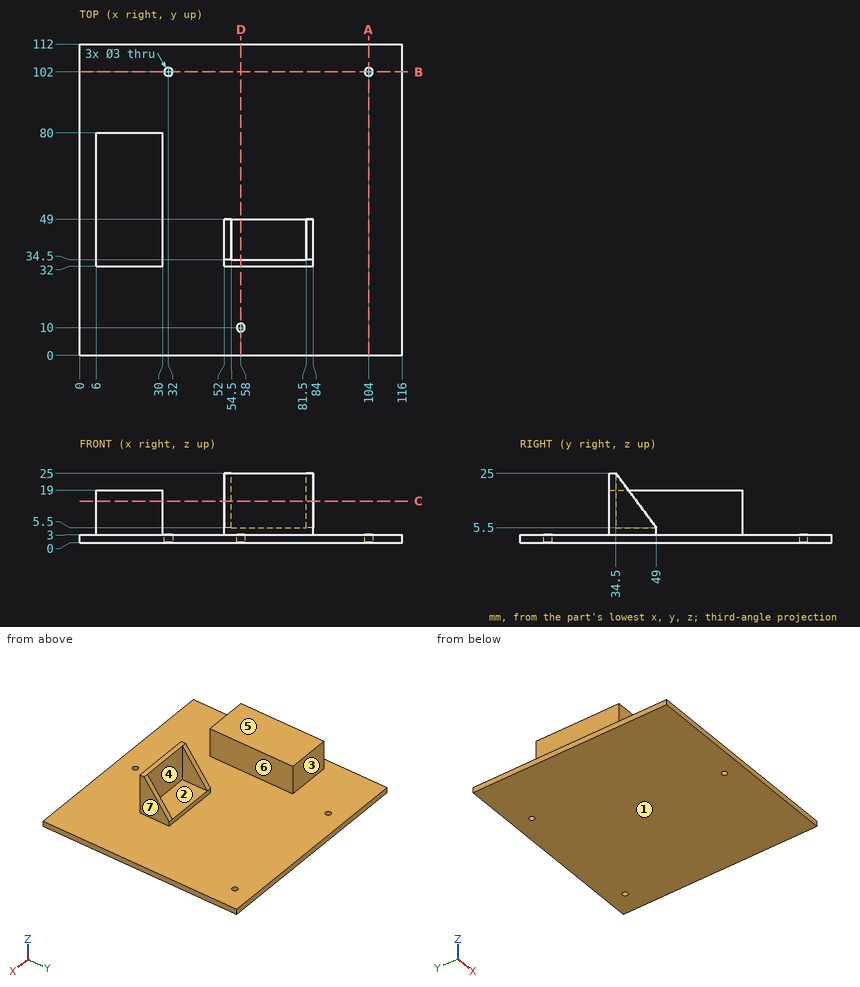
Study the drawing (mm; zero at the part's minimum x, y, z) and answer. A direction names the side the tool comes from. Give positions to 0.01 mm unless a question says otherwise; leave off trailing zeros. Write each loop counter-clockwise with the first axis right and the second up, starting at its lowest first coordinate (ties: lowest second). Pieces come first, ordered by that corner, then holes.
Item 1: Section A-A, the plane x = 104 is taken. Write down the section's boundary in (y, z).
Item 2: Section C-C, the plane z = 15 is taken. Write down the section's boundary in (x, y), plus the area to 3 significant figures.
Item 3: Section D-D, the plane x = 58 is taken. Write down the section's boundary in (y, z).
Item 4: Determine the mould class of the marked faces 4, 5, 6 and 7 for opening direction X: released by +X, released by -X, zero draft, split by the parting line, or undercut.
Item 5: Section B-B, the plane y = 102 is taken. Write down the section's boundary in (x, z), plus the area to 3 significant figures.
Item 6: Which of the six approach directions +Z, -Z, +X, -X, +Y, -Y give full straight-line access (tool end or side, diameter ignored) to the marked faces 1, 2 and 3?
Item 7: Flat-ended cylindrical pins translate along their axes: P1, Ø6, axis at x = 63, z = 12.5, coming from the +Y side; P2, Ø5, axis at x = 15, z = 10, coming from the +Y side; P3, Ø5, axis at y = 38.5, z = 10, coming from the +X side. Find the tip coordinate at first contact, or state that the pin passes through.
Item 8: Find the intervals of material crossed by line 1 along X through (y, z) = (102, 1.9); line 2 along X through (y, z) = (45.5, 9.5); line 3 along X through (y, z) = (44, 4.75), in increasing order.
Completed:
1. outline: (0, 0) - (100.5, 0) - (100.5, 3) - (0, 3) - close; (103.5, 0) - (112, 0) - (112, 3) - (103.5, 3) - close
2. outline: (6, 32) - (30, 32) - (30, 80) - (6, 80) - close; (52, 32) - (84, 32) - (84, 41.94) - (81.5, 41.94) - (81.5, 34.5) - (54.5, 34.5) - (54.5, 41.94) - (52, 41.94) - close
2. area: 1,270 mm2
3. outline: (0, 0) - (8.5, 0) - (8.5, 3) - (0, 3) - close; (11.5, 0) - (112, 0) - (112, 3) - (49, 3) - (49, 5.5) - (34.5, 5.5) - (34.5, 25) - (32, 25) - (32, 3) - (11.5, 3) - close
4. face 4: undercut
4. face 5: zero draft
4. face 6: undercut
4. face 7: released by +X
5. outline: (0, 0) - (30.5, 0) - (30.5, 3) - (0, 3) - close; (33.5, 0) - (102.5, 0) - (102.5, 3) - (33.5, 3) - close; (105.5, 0) - (116, 0) - (116, 3) - (105.5, 3) - close
5. area: 330 mm2
6. face 1: -Z, +X, -X, +Y, -Y
6. face 2: +Z, +Y
6. face 3: +Z, +X, -X, +Y
7. P1: stops at y = 34.5
7. P2: stops at y = 80
7. P3: stops at x = 84
8. line 1: x = 0 to 30.5, 33.5 to 102.5, 105.5 to 116
8. line 2: x = 6 to 30, 52 to 54.5, 81.5 to 84
8. line 3: x = 6 to 30, 52 to 84
